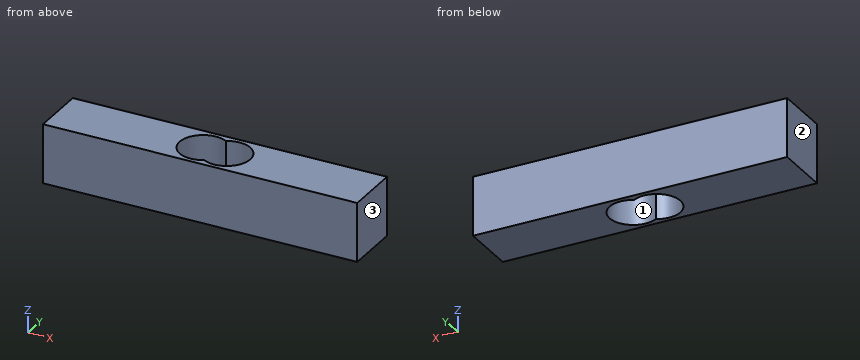
```python
from build123d import *

# Parameters (mm, degrees)
SKETCH1_W           = 80
SKETCH1_H           = 15
BOSS_EXTRUDE1_DEPTH = 14.2
CUT_EXTRUDE1_DEPTH  = 46.018218534


with BuildPart() as part:
    # Sketch1 → Boss-Extrude1 (new body)
    with BuildSketch(Plane(origin=(0, 0, 0), x_dir=(1, 0, 0), z_dir=(0, 1, 0))):
        Rectangle(SKETCH1_W, SKETCH1_H)
    extrude(amount=BOSS_EXTRUDE1_DEPTH)

    # Sketch4 → Cut-Extrude1 (cut, through all)
    with BuildSketch(Plane.XY.offset(7.5)):
        with BuildLine():
            ThreePointArc((0, 1.903847577), (9, 7.1), (0, 12.296152423))
            ThreePointArc((0, 12.296152423), (-9, 7.1), (0, 1.903847577))
        make_face()
    extrude(amount=-CUT_EXTRUDE1_DEPTH, mode=Mode.SUBTRACT)


solid = part.part
```
Geometry check sheet. Reference: the model listing, model coordinates, mm. Face numbers are marked on the shaded views. Give positions to 0.01 mm unless a question says otherwise; leave off trailing zeros. Write each loop counter-clockwise with the first axis right and the second up, starting at its lowest first coordinate (ties: lowest second). Pieces come first, ordered by that corner, then holes.
1) Section check B-B, the plane x = 3. Record the boundary of the cut face in (y, z), and give its area (3 significant figures).
2) Release check for a two-part mould opening along X. For the marked faces 1, 2 and 3 record: pulls with the +X half, pulls with the -X half, needs draft (parallel to the pull), parting line crosses it, or undercut.
3) Section check C-C, the plane z = 5.5. Record the boundary of the cut face in (x, y).
4) Gauge pin test, flat end, axial feed: pin 1 (7 mm diameter, centred on x = 3, y = 7.1, fed in from -Z). Record the tip position at first contact, or that the pin passes through.
5) Material ranges on L1, parallel to Y at x = 3, z = 2.75; L2, parallel to X at y = 7, z = -4.5; L3, parallel to X at y = 4.5, z = -3.75, recorded low to high.
6) Section check A-A, the plane y = 7.1. Record the boundary of the cut face in (x, z).
Computed:
1. outline: (0, -7.5) - (1.1, -7.5) - (1.1, 7.5) - (0, 7.5) - close; (13.1, -7.5) - (14.2, -7.5) - (14.2, 7.5) - (13.1, 7.5) - close
1. area: 33.0 mm2
2. face 1: undercut
2. face 2: pulls with the -X half
2. face 3: pulls with the +X half
3. outline: (-40, 0) - (40, 0) - (40, 14.2) - (-40, 14.2) - close; hole (0, 1.9) arc R6 ccw (long way) to (0, 12.3) arc R6 ccw (long way) to start
4. pin 1: passes through
5. L1: y = 0 to 1.1, 13.1 to 14.2
5. L2: x = -40 to -9, 9 to 40
5. L3: x = -40 to -8.41, 8.41 to 40
6. outline: (-40, -7.5) - (-9, -7.5) - (-9, 7.5) - (-40, 7.5) - close; (9, -7.5) - (40, -7.5) - (40, 7.5) - (9, 7.5) - close
